Answer from the drawing. Dimensions are ordinates in mm from the lowest x, y and z of the part. Give positions to 0.01 mm unless a question says otherwise; leave off trailing zeros. Loops run counter-clockwise (first coordinate to the right, second up) from the corner with the lowest first, then second, coordinate; pieces in that order, holes last. Notation, with made-up numbers: (63, 27) - (71, 27) arc R17 cw to (71, 42) - close; hole circle Ø11 at (42.25, 9). An arc over 180 degrees is marked (long way). Put each result on its own line as item: value. Start each with the question number.
1. A cutting plane is placed at A-A, the plane z = 289. Determine the outline of the cut face in (x, y), plus the area to 3 significant figures.
2. Given pin 1 Ø8 at (x, z) = (153.5, 322) entering from +Y; pin 2 Ø2.5 at (y, z) = (2, 75.5) entering from -X, each flat-ended and moving along its own axis, determine where each tip first touches the part or whether it passes through.
3. Consider L1, parallel to X at y = 7, z = 113.5; L2, parallel to Y at x = 178, z = 290; L3, parallel to X at y = 3.5, z = 29. Determine where each line is inside the solid, lowest interval first. Write a range as from..to.
4. A cutting plane is placed at C-C, the plane x = 97. Determine the outline of the cut face in (y, z), plus the area to 3 significant figures.
5. A cutting plane is placed at B-B, the plane x = 130. Determine the outline of the cut face in (y, z).
6. For a pull along X with two mould halves and no side action, classify the marked faces 1 and 2 as released by +X, released by -X, zero draft, split by the parting line, or undercut.
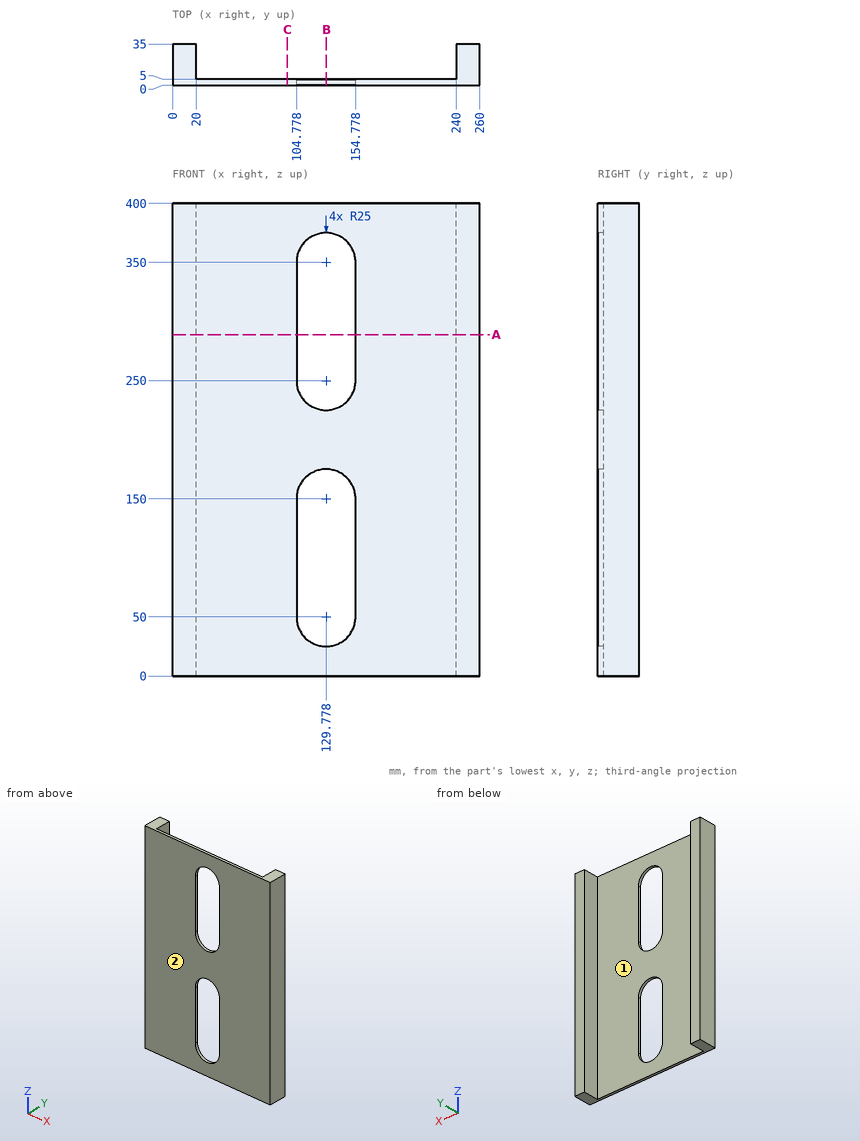
Return value:
1. outline: (0, 0) - (104.78, 0) - (104.78, 5) - (20, 5) - (20, 35) - (0, 35) - close; (154.78, 0) - (260, 0) - (260, 35) - (240, 35) - (240, 5) - (154.78, 5) - close
1. area: 2,250 mm2
2. pin 1: stops at y = 5
2. pin 2: stops at x = 0
3. L1: x = 0..20, 240..260
3. L2: y = 0..5
3. L3: x = 0..116.21, 143.34..260
4. outline: (0, 0) - (5, 0) - (5, 400) - (0, 400) - close
4. area: 2,000 mm2
5. outline: (0, 0) - (5, 0) - (5, 25) - (0, 25) - close; (0, 175) - (5, 175) - (5, 225) - (0, 225) - close; (0, 375) - (5, 375) - (5, 400) - (0, 400) - close
6. face 1: undercut
6. face 2: zero draft
